from build123d import *

# Parameters (mm, degrees)
SKETCH_W     = 80
SKETCH_H     = 30
SKETCH_R     = 2
SKETCH_W_2   = 8.5
SKETCH_H_2   = 5
SKETCH_W_3   = 30.5
SKETCH_H_3   = 10
PAD_DEPTH    = 3
SKETCH002_W  = 8
SKETCH002_H  = 5
PAD001_DEPTH = 29
SKETCH003_R  = 1.5
POCKET_DEPTH = 30.001


with BuildPart() as part:
    # Sketch → Pad (new body)
    with BuildSketch(Plane.XY):
        with Locations((40, 15)):
            Rectangle(SKETCH_W, SKETCH_H)
        with Locations((3, 27)):
            Circle(SKETCH_R, mode=Mode.SUBTRACT)
        with Locations((77, 27)):
            Circle(SKETCH_R, mode=Mode.SUBTRACT)
        with Locations((77, 3)):
            Circle(SKETCH_R, mode=Mode.SUBTRACT)
        with Locations((3, 3)):
            Circle(SKETCH_R, mode=Mode.SUBTRACT)
        with Locations((56.75, 13)):
            Rectangle(SKETCH_W_2, SKETCH_H_2, mode=Mode.SUBTRACT)
        with Locations((32.25, 14)):
            Rectangle(SKETCH_W_3, SKETCH_H_3, mode=Mode.SUBTRACT)
    extrude(amount=PAD_DEPTH)

    # Sketch002 (on Sketch) → Pad001 (join)
    with BuildSketch(Plane(origin=(0, 0, 0), x_dir=(1, 0, 0), z_dir=(0, 0, -1))):
        with Locations((11.5, -10)):
            Rectangle(SKETCH002_W, SKETCH002_H)
        with Locations((68.5, -10)):
            Rectangle(SKETCH002_W, SKETCH002_H)
    extrude(amount=PAD001_DEPTH)

    # Sketch003 → Pocket (cut, through all)
    with BuildSketch(Plane.XZ):
        with Locations((11.5, -4.5)):
            Circle(SKETCH003_R)
        with Locations((68.5, -4.5)):
            Circle(SKETCH003_R)
        with Locations((11.5, -25.5)):
            Circle(SKETCH003_R)
        with Locations((68.5, -25.5)):
            Circle(SKETCH003_R)
    extrude(amount=-POCKET_DEPTH, mode=Mode.SUBTRACT)


solid = part.part
Geometry check sheet. Reference: the model listing, model coordinates, mm. A direction names the side the tool comes from. Coordinates: 2 decimals unless noted, no trailing zeros. Loops run counter-clockwise (first coordinate to the right, second up) from the corner with the lowest first, then second, coordinate; pieces in that order, holes last. Notation, with made-up numbers: (29, 85.5) - (42, 85.5) arc R32 cw to (42, 111.5) - close; hole circle Ø6 at (-13, 46.5). An arc over 180 degrees is marked (long way). Use one line per item in the form item = value. Start each with the question number.
Item 1: Gauge pin test, flat ends, axial feed: pin 1 (3.5 mm diameter, centred on x = 68.5, z = -25.5, fed in from -Y); pin 2 (1 mm diameter, centred on x = 72, z = -13.5, fed in from +Y); pin 3 (9 mm diameter, centred on x = 45, y = 21.5, fed in from -Z). Record the tip position at first contact, or that the pin passes through.
Item 2: Section check B-B, the plane y = 17.5. Enter the section's corners in (x, z), and give its area (4 significant figures).
Item 3: Mould release check, pull along X, two halves, no side actions. Record for faces 1 (the face through (72.5, 10, -14)), 2 (the face through (7.5, 10, -14)), 3 (the face through (77.923, 25.226, 1.479)): +X half, -X half, draft (parallel to the pull), parting line (faces both ways), or undercut.
Item 4: Section check C-C, the plane x = 11.5. Enter the section's corners in (y, z).
Item 5: Tool access check on faces 4 (the face through (11, 12.5, -14)), 5 (the face through (57, 15.5, 1)), 6 (the face through (11, 7.5, -14)), 7 (the face through (15.5, 10, -14)). Record the directions out of +Z, -Z, +X, -X, +Y, -Y that give a thin tool (end or side, any length) a straight path to the whole face; none if there is none.
Item 6: Section check A-A, the plane z = -25.5. Enter the section's corners in (x, y).
Item 7: Section check D-D, the plane y = 27. Enter the section's corners in (x, z), and give its area (3 significant figures).
Item 8: Thickness scan on probe 1 along Z at (x, y) = (11.5, 10.85); probe 2 along Z at (x, y) = (69, 8.5); probe 3 along Z at (x, y) = (19, 1.75). Record the ranges inside material, lowest first.
Computed:
q1.pin_1 = 7.5
q1.pin_2 = 12.5
q1.pin_3 = 0
q2.outline = (0, 0) - (17, 0) - (17, 3) - (0, 3) - close; (47.5, 0) - (80, 0) - (80, 3) - (47.5, 3) - close
q2.area = 148.5 mm2
q3.face_1 = +X half
q3.face_2 = -X half
q3.face_3 = undercut
q4.outline = (0, 0) - (7.5, 0) - (7.5, -3) - (12.5, -3) - (12.5, 0) - (30, 0) - (30, 3) - (0, 3) - close; (7.5, -29) - (12.5, -29) - (12.5, -27) - (7.5, -27) - close; (7.5, -24) - (12.5, -24) - (12.5, -6) - (7.5, -6) - close
q5.face_4 = -Z, +X, -X, +Y
q5.face_5 = +Z, -Z
q5.face_6 = -Z, +X, -X, -Y
q5.face_7 = -Z, +Y, -Y
q6.outline = (7.5, 7.5) - (10, 7.5) - (10, 12.5) - (7.5, 12.5) - close; (13, 7.5) - (15.5, 7.5) - (15.5, 12.5) - (13, 12.5) - close; (64.5, 7.5) - (67, 7.5) - (67, 12.5) - (64.5, 12.5) - close; (70, 7.5) - (72.5, 7.5) - (72.5, 12.5) - (70, 12.5) - close
q7.outline = (0, 0) - (1, 0) - (1, 3) - (0, 3) - close; (5, 0) - (75, 0) - (75, 3) - (5, 3) - close; (79, 0) - (80, 0) - (80, 3) - (79, 3) - close
q7.area = 216 mm2
q8.probe_1 = -29 to -27, -24 to -6, -3 to 3
q8.probe_2 = -29 to -26.91, -24.09 to -5.91, -3.09 to 3
q8.probe_3 = 0 to 3
